from build123d import *

# Parameters (mm, degrees)
SCREW_HOLES_COUNT = 12


with BuildPart() as part:
    # Cross Section → Main (revolve)
    with BuildSketch(Plane.XY):
        Polygon((-38.1, 0), (-38.1, -3.175), (-38.8874, -3.175), (-38.8874, -15.875), (-39.68115, -15.875), (-39.68115, -3.175), (-46.53915, -3.175), (-46.53915, 9.525), (-45.72, 9.525), (-45.72, 0), align=None)
    revolve(axis=Axis((0, 55, 0), (0, -1, 0)))

    # Sketch7 → #3-48 Tapped Hole1 (revolve, cut)
    with BuildSketch(Plane(origin=(-42.700575, 0, 0), x_dir=(0, 0, 1), z_dir=(1, 0, 0))):
        Polygon((0, 0), (0, 3.901027994), (0.99695, 3.302), (0.99695, 0), align=None)
    f_3_48_tapped_hole1 = revolve(axis=Axis((-42.700575, 6.35, 0), (0, -1, 0)), mode=Mode.SUBTRACT)

    # Screw Holes: #3-48 Tapped Hole1 ×12 about axis
    screw_holes_axis = Axis((0, 0, 0), (0, 1, 0))
    for i in range(1, SCREW_HOLES_COUNT):
        add(f_3_48_tapped_hole1.rotate(screw_holes_axis, i * 360 / SCREW_HOLES_COUNT), mode=Mode.SUBTRACT)


solid = part.part
Input: part model. Units: mm. Frame: model coordinates. A direction names the side the tool comes from. Round coordinates to 2 decimals unless told otherwise and drop trailing zeros. Order: outer loops, then holes, each group sorted by start corner. A loop starts at its lowest first (then second) coordinate and runs counter-clockwise, first axis right, second up. Notation, with made-up numbers: (25, -33) - (69, -33) arc R27 ccw to (69, 5) - close; hole circle Ø4 at (-24, -1). An arc over 180 degrees is marked (long way). Answer as a JSON object with one key per item and string values. Group by question number.
(1) Material intervals for probe 1 along X at (y, z) = (-1.4, 0); probe 2 along X at (y, z) = (-7.5, 0), sorted ascending. Write a range as from..to.
(2) Cut plane C-C (y = 6.5). Return loops of the section in (x, z).
(3) Reachability of faces 4 (the face through (-43.61, 4.7, -13.73)), 5 (the face through (25.7, -3.175, 28.6)), 6 (the face through (36.93, 3.26, 28.32)) from +Z, -Z, +X, -X, +Y, -Y: full face, straight path, thin tool, end or side. Return the list, or none.
(4) Cut plane A-A (x = -26). Return loops of the section in (y, z) (3 decimals).
(5) Cut plane B-B (z = -29). Return loops of the section in (x, y) (3 decimals).
(6) Cut plane D-D (y = -5.75). Return loops of the section in (x, z), then the cut area to 3 significant figures.
(7) Pin query (flat end, axial travel): P1, Ø2.5, axis at x = 0, z = 42.7, coming from the -Y side (3 decimals); P2, Ø4, axis at y = -0.5, z = 20.5, coming from the +X side; P3, Ø10, axis at y = -11.5, z = -1.5, coming from the -X side. Return the tip coordinate at first contact, or that it passes through.
(8) Draft query along X for faces 1 (the face through (26.3, -15.875, 29.2)), 2 (the face through (5.166, -9.436, -39.343)), 3 (the face through (27.3, 0, -27.3)). Return one class per face: released by +X, released by -X, zero draft, split by the parting line, or undercut.
Here are the results:
{
 "1": {"probe 1": "x = -46.54..-43.7, -41.7..-38.1, 38.1..41.7, 43.7..46.54", "probe 2": "x = -39.68..-38.89, 38.89..39.68"},
 "2": {"outline": "circle Ø93.08 at (0, 0); hole circle Ø91.44 at (0, 0)"},
 "3": {"face 4": "+Y", "face 5": "-Y", "face 6": "+Y, -Y"},
 "4": {"outline": "(-15.875, -29.977) - (-3.175, -29.977) - (-3.175, -38.599) - (9.525, -38.599) - (9.525, -37.607) - (0, -37.607) - (0, -27.85) - (-3.175, -27.85) - (-3.175, -28.918) - (-15.875, -28.918) - close; (-15.875, 28.918) - (-3.175, 28.918) - (-3.175, 27.85) - (0, 27.85) - (0, 37.607) - (9.525, 37.607) - (9.525, 38.599) - (-3.175, 38.599) - (-3.175, 29.977) - (-15.875, 29.977) - close"},
 "5": {"outline": "(-36.399, -3.175) - (-27.085, -3.175) - (-27.085, -15.875) - (-25.908, -15.875) - (-25.908, -3.175) - (-24.711, -3.175) - (-24.711, 0) - (-35.346, 0) - (-35.346, 9.525) - (-36.399, 9.525) - close; (24.711, -3.175) - (25.908, -3.175) - (25.908, -15.875) - (27.085, -15.875) - (27.085, -3.175) - (36.399, -3.175) - (36.399, 9.525) - (35.346, 9.525) - (35.346, 0) - (24.711, 0) - close"},
 "6": {"outline": "circle Ø79.36 at (0, 0); hole circle Ø77.77 at (0, 0)", "area": "196 mm^2"},
 "7": {"P1": "stops at y = -3.175", "P2": "stops at x = 42.7", "P3": "stops at x = -39.68"},
 "8": {"face 1": "zero draft", "face 2": "split by the parting line", "face 3": "undercut"}
}
